Check sheet for the drawn part. Datum: minimum x, y, z corner. Units: mm. Round coordinates to 2 decimals unless told otherwise and drop trailing zeros. Write each loop counter-clockwise with the first axis right and the second up, starting at its lowest first coordinate (ties: lowest second). Pieces come first, ordered by that corner, then holes. Notation, with made-up numbers: M -25.5,42 L 5.5,42 A7 cw 5.5,46 Z; hole C -9.75,-37.75 d3. An arc over 180 degrees is marked long. Put each result on its own line as item: value.
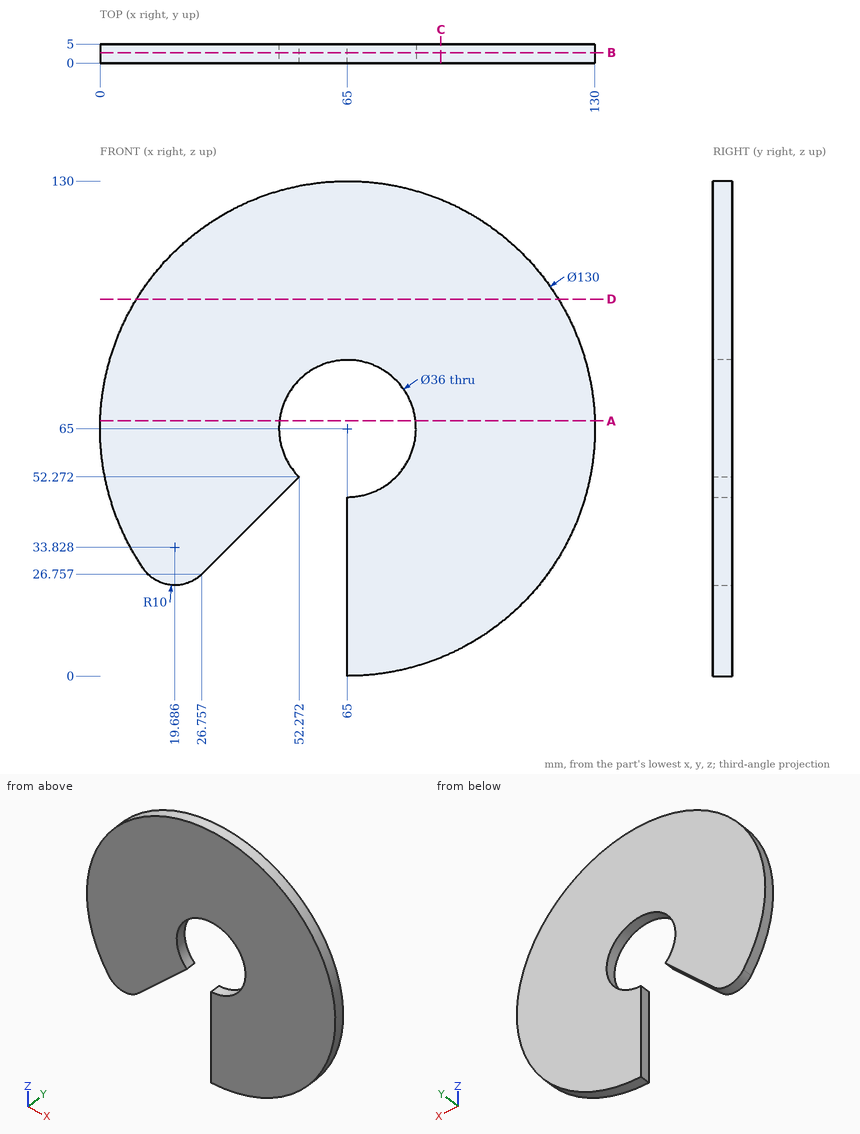
1. Cross-section at D-D (z = 99). Enter the section's corners in (x, y).
Computed values:
outline: M 9.6,0 L 120.4,0 L 120.4,5 L 9.6,5 Z
2. Depth check by flat-ended pin: pin 1 Ø1.5 at (x, y) = (53, 3.5) entering from +Z; pin 2 Ø2 at (y, z) = (4, 47.5) entering from -X; pin 3 Ø2.5 at (y, z) = (2, 35) entering from -X. Enter the tip coordinate at first touch or a pass-through.
Computed values:
pin 1: stops at z = 129.02
pin 2: stops at x = 2.13
pin 3: stops at x = 6.7
3. Cross-section at B-B (y = 2.75). Enter the section's corners in (x, z).
Computed values:
outline: M 11.45,28.16 A10 ccw 26.76,26.76 L 52.27,52.27 A18 cw long 65,47 L 65,0 A65 ccw long Z
4. Cross-section at C-C (x = 89.5). Enter the section's corners in (y, z), then the cut area to 3 significant figures.
Computed values:
outline: M 0,4.79 L 5,4.79 L 5,125.21 L 0,125.21 Z
area: 602 mm2
5. Scan lines: probe 1 along X at (y, z) = (3.35, 65); probe 2 along X at (y, z) = (1.15, 40); probe 3 along X at (y, z) = (3.8, 17). Record each from-to range of solid material in increasing order.
Computed values:
probe 1: x = 0 to 47, 83 to 130
probe 2: x = 5 to 40, 65 to 125
probe 3: x = 65 to 108.83
6. Cross-section at A-A (z = 67). Enter the section's corners in (x, y).
Computed values:
outline: M 0.03,0 L 47.11,0 L 47.11,5 L 0.03,5 Z; M 82.89,0 L 129.97,0 L 129.97,5 L 82.89,5 Z
